Geometry check sheet. Reference: the model listing, model coordinates, mm. Face numbers are marked on the shaded views. A direction names the side the tool comes from. Give positions to 0.01 mm unless a question says otherwise; leave off trailing zeros. Write each loop counter-clockwise with the first axis right and the second up, starting at its lowest first coordinate (ties: lowest second). Pieces come first, ordered by that corner, then holes. Notation, with made-up numbers: (16, 33.25) -> (63, 33.25) arc R28 ccw to (63, 65.25) -> close; hole circle Ø1 at (-7, -28.5). An arc over 180 degrees is marked (long way). Use a Markdown table: item, result. Add a question column.
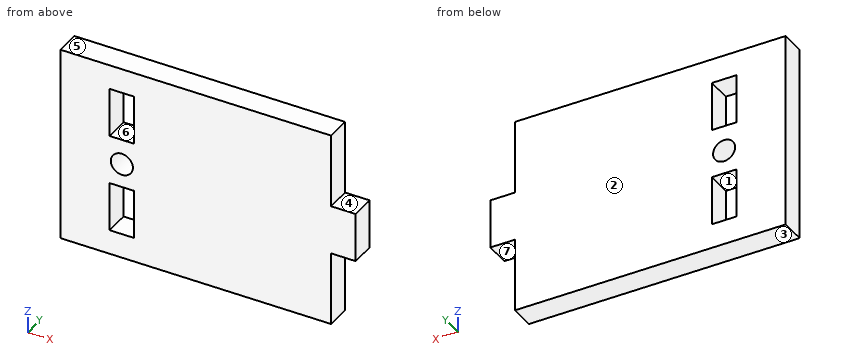
from build123d import *

# Parameters (mm, degrees)
SKETCH1_R           = 2.846646533
SKETCH1_W           = 6.35
SKETCH1_H           = 12.7
BOSS_EXTRUDE1_DEPTH = 6.35


with BuildPart() as part:
    # Sketch1 → Boss-Extrude1 (new body)
    with BuildSketch(Plane(origin=(0, 0, 0), x_dir=(1, 0, 0), z_dir=(0, 1, 0))):
        Polygon((0, 0), (69.85, 0), (69.85, 19.05), (76.2, 19.05), (76.2, 31.75), (69.85, 31.75), (69.85, 50.8), (0, 50.8), align=None)
        with Locations((15.875, 25.640429005)):
            Circle(SKETCH1_R, mode=Mode.SUBTRACT)
        with Locations((15.875, 38.1)):
            Rectangle(SKETCH1_W, SKETCH1_H, mode=Mode.SUBTRACT)
        with Locations((15.875, 12.7)):
            Rectangle(SKETCH1_W, SKETCH1_H, mode=Mode.SUBTRACT)
    extrude(amount=BOSS_EXTRUDE1_DEPTH)


solid = part.part
1) Sectioned sample at C-C, the plane y = 3.25. Enter the section's corners in (x, z) (3 decimals).
2) Draft check along X on the marked faces 1 and 2. Enter one of: +X half, -X half, draft (parallel to the pull), parting line (faces both ways), or undercut.
3) Sectioned sample at A-A, the plane x = 14. Enter the section's corners in (y, z), and give its area (3 significant figures).
4) Material ranges on probe 1 along X at (y, z) = (0.5, -39.5); probe 2 along Z at (x, y) = (13.5, 3); probe 3 along Z at (x, y) = (15, 5), recorded low to high. Write a range as [from, to].
5) Gauge pin test, flat ends, axial feed: P1, Ø3, axis at x = 72.5, y = 2, coming from the +Z side; P2, Ø3, axis at y = 4.5, z = -15, coming from the +X side. Record the tip position at first contact, or that the pin passes through.
6) Tool access check on the marked faces 3, 4, 5, 6 and 7. Record the directions out of +Z, -Z, +X, -X, +Y, -Y that give a thin tool (end or side, any length) a straight path to the whole face; none if there is none.
7) Sectioned sample at B-B, the plane z = -10.5. Enter the section's corners in (x, y), and give its area (3 significant figures).
Check values:
| question | item | result |
|---|---|---|
| 1 | outline | (0, -50.8) -> (69.85, -50.8) -> (69.85, -31.75) -> (76.2, -31.75) -> (76.2, -19.05) -> (69.85, -19.05) -> (69.85, 0) -> (0, 0) -> close; hole (12.7, -44.45) -> (19.05, -44.45) -> (19.05, -31.75) -> (12.7, -31.75) -> close; hole (12.7, -19.05) -> (19.05, -19.05) -> (19.05, -6.35) -> (12.7, -6.35) -> close; hole circle Ø5.693 at (15.875, -25.64) |
| 2 | face 1 | undercut |
| 2 | face 2 | draft |
| 3 | outline | (0, -50.8) -> (6.35, -50.8) -> (6.35, -44.45) -> (0, -44.45) -> close; (0, -31.75) -> (6.35, -31.75) -> (6.35, -27.78) -> (0, -27.78) -> close; (0, -23.5) -> (6.35, -23.5) -> (6.35, -19.05) -> (0, -19.05) -> close; (0, -6.35) -> (6.35, -6.35) -> (6.35, 0) -> (0, 0) -> close |
| 3 | area | 134 mm² |
| 4 | probe 1 | [0, 12.7], [19.05, 69.85] |
| 4 | probe 2 | [-50.8, -44.45], [-31.75, -27.21], [-24.07, -19.05], [-6.35, 0] |
| 4 | probe 3 | [-50.8, -44.45], [-31.75, -28.35], [-22.93, -19.05], [-6.35, 0] |
| 5 | P1 | z = -19.05 |
| 5 | P2 | x = 69.85 |
| 6 | face 3 | -Z, +X, -X, +Y, -Y |
| 6 | face 4 | +Z, +X, +Y, -Y |
| 6 | face 5 | +Z, +X, -X, +Y, -Y |
| 6 | face 6 | +Y, -Y |
| 6 | face 7 | -Z, +X, +Y, -Y |
| 7 | outline | (0, 0) -> (12.7, 0) -> (12.7, 6.35) -> (0, 6.35) -> close; (19.05, 0) -> (69.85, 0) -> (69.85, 6.35) -> (19.05, 6.35) -> close |
| 7 | area | 403 mm² |
